Can you work these out from the model? Positions are in its coordinate system, mm. A direction names the side the tool comes from. Round coordinates to 2 decimals unless told otherwise and drop trailing zeros. Loops run counter-clockwise (first coordinate to the right, second up) from the corner with the lowest first, then second, coordinate; pieces in that order, holes last.
```python
from build123d import *

# Parameters (mm, degrees)
F1_DEPTH = 63.5
F2_DEPTH = 25.4
F3_DEPTH = 7.9375
F0_W     = 27.708321
F0_H     = 19.05
F4_DEPTH = 25.4
F6_R     = 6.35


with BuildPart() as f1:
    # F0 (on Front) → F1 (new body, symmetric)
    with BuildSketch(Plane.XZ):
        Polygon((41.275, -9.525), (41.275, 9.525), (22.225, 9.525), (-41.275, 9.525), (-41.275, -9.525), align=None)
    extrude(amount=F1_DEPTH, both=True)

    # F0 (on Front) → F2 (join, symmetric)
    with BuildSketch(Plane.XZ):
        with BuildLine():
            Line((22.225, 9.525), (41.275, 9.525))
            Line((41.275, 9.525), (41.275, 27.0002))
            ThreePointArc((41.275, 27.0002), (45.92468, 38.22552), (57.15, 42.8752))
            Line((57.15, 42.8752), (60.325, 42.8752))
            Line((60.325, 42.8752), (60.325, 61.9252))
            add(Edge.make_bspline(
                [(50.978388, 61.375581), (54.16985, 61.649544), (57.295356, 61.833243), (60.325, 61.9252)],
                knots=[106.038732, 106.038732, 106.038732, 106.038732, 114.316845, 114.316845, 114.316845, 114.316845], degree=3))
            ThreePointArc((50.978388, 61.375581), (30.361017, 49.407923), (22.225, 27.0002))
            Line((22.225, 27.0002), (22.225, 9.525))
        make_face()
    extrude(amount=F2_DEPTH, both=True)

    # F0 (on Front) → F3 (join, symmetric)
    with BuildSketch(Plane.XZ):
        with BuildLine():
            Line((-41.275, 9.525), (22.225, 9.525))
            Line((22.225, 9.525), (22.225, 27.0002))
            ThreePointArc((22.225, 27.0002), (30.361017, 49.407923), (50.978388, 61.375581))
            add(Edge.make_bspline(
                [(-41.275, 9.525), (-41.606238, 39.546193), (10.097253, 57.86625), (50.978388, 61.375581)],
                knots=[0, 0, 0, 0, 106.038732, 106.038732, 106.038732, 106.038732], degree=3))
        make_face()
    extrude(amount=F3_DEPTH, both=True)

    # F0 (on Front) → F4 (join, symmetric)
    with BuildSketch(Plane.XZ):
        with Locations((74.17916, 52.4002)):
            Rectangle(F0_W, F0_H)
    extrude(amount=F4_DEPTH, both=True)

    # F0 (on Front) → F5 (revolve)
    with BuildSketch(Plane.XZ):
        Polygon((88.033321, 61.9252), (88.033321, 42.8752), (88.033321, 38.1), (111.125, 38.1), (111.125, 66.675), (88.033321, 66.675), align=None)
    revolve(axis=Axis((88.033321, 0, 52.3875), (0, 0, -1)))

    # F6
    f6_edges = [f1.edges().sort_by_distance(p)[0] for p in [
        (41.275, -63.5, 0),
        (-41.275, -63.5, 0),
        (-41.275, 63.5, 0),
        (41.275, 63.5, 0),
    ]]
    fillet(f6_edges, radius=F6_R)


solid = f1.part
```
(1) For pin 1 (6 mm diameter, centred on y = -25, z = 11, fed in from +X) (3 decimals); pin 2 (2.5 mm diameter, centred on y = 24.5, z = 50.5, fed in from +X); pin 3 (5 mm diameter, centred on x = 2.5, z = 56, fed in from -Y) (3 decimals); pin 4 (1 mm diameter, centred on y = 14.5, z = 34, fed in from +X), each with a flat end and sliding along its axis, tell me the tip position at first contact or that it passes through.
(2) Suppose I cut it at D-D (x = 91). Write out the boundary of the cut face in (y, z) (3 decimals).
(3) Suppose I cut it at C-C (y = 34.5). Write out the boundary of the cut face in (x, z) (3 decimals).
(4) Which directions (+Z, -Z, +X, -X, +Y, -Y) give clear straight access to the entire face, cutting with the end or side of a thin tool? Please do faces 1 (the flat face through (41.275, -1, 4)), 2 (the cylindrical face through (30.58, 16.55, 49.67)), 3 (the flat face through (47, -25.4, 42)), 4 (the flat face through (47, 25.4, 42)).
(5) Suppose I cut it at A-A (z = 5.5). Write out the boundary of the cut face in (x, y) (3 decimals).
(6) If I drill on line 1 (X direction, y = 9, z = 14) (3 decimals); line 2 (X direction, y = -22.5, z = -6) (3 decimals); line 3 (Y direction, x = 41, z = 53.5), over which ranges is the centre line in solid material (lowest first)?
(7) Suppose I cut it at B-B (x = 68.5). Write out the boundary of the cut face in (y, z) (3 decimals), then the cut area to 3 significant figures.
Check result:
1. pin 1: stops at x = 41.275
1. pin 2: stops at x = 88.03
1. pin 3: passes through
1. pin 4: stops at x = 43.16
2. outline: (-22.9, 38.1) - (22.9, 38.1) - (22.9, 66.675) - (-22.9, 66.675) - close
3. outline: (-41.275, -9.525) - (41.275, -9.525) - (41.275, 9.525) - (-41.275, 9.525) - close
4. face 1: -Z, +X, +Y, -Y
4. face 2: +Z, -X, +Y
4. face 3: +Z, +X, -X, -Y
4. face 4: +Z, +X, -X, +Y
5. outline: (-41.275, -57.15) arc R6.35 ccw to (-34.925, -63.5) - (34.925, -63.5) arc R6.35 ccw to (41.275, -57.15) - (41.275, 57.15) arc R6.35 ccw to (34.925, 63.5) - (-34.925, 63.5) arc R6.35 ccw to (-41.275, 57.15) - close
6. line 1: x = 22.225 to 41.275
6. line 2: x = -41.275 to 41.275
6. line 3: y = -25.4 to 25.4
7. outline: (-25.4, 42.875) - (-12.316, 42.875) - (-12.316, 38.1) - (12.316, 38.1) - (12.316, 42.875) - (25.4, 42.875) - (25.4, 61.925) - (12.316, 61.925) - (12.316, 66.675) - (-12.316, 66.675) - (-12.316, 61.925) - (-25.4, 61.925) - close
7. area: 1,200 mm2
